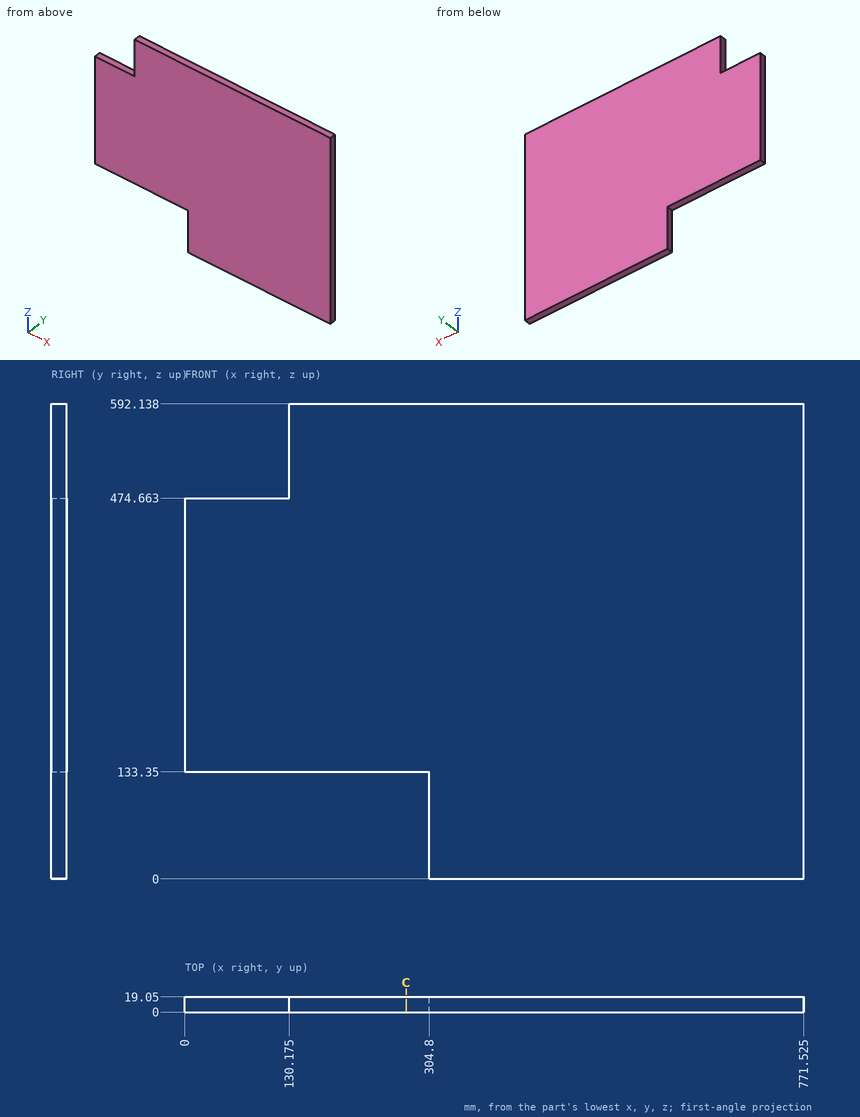
Can you work these out from the drawing? Everything is in mm from the part's minimum corner. Round coordinates to 2 decimals unless told otherwise and drop trailing zeros. Order: outer loops, then holes, each group sorted by start corner. A loop starts at its lowest first (then second) coordinate and runs counter-clockwise, first axis right, second up.
(1) I'm going to push flat-ended pins straight in: pin 1 (4 mm diameter, centred on x = 201, z = 344, fed in from -Y); pin 2 (2 mm diameter, centred on x = 109, y = 8, fed in from +Z). Where does each tip first touch, or does it pass through?
Results are:
pin 1: stops at y = 0
pin 2: stops at z = 474.66
(2) If I drill on L1, parallel to Z at x = 288.5, y = 4.75; L2, parallel to X at y = 13, z = 49 (1 decimal), over which ranges is the centre line in solid material (lowest first)?
Results are:
L1: z = 133.35 to 592.14
L2: x = 304.8 to 771.5
(3) If we section it at C-C (x = 276): Please give me the cut outline in (y, z).
Results are:
outline: (0, 133.35) - (19.05, 133.35) - (19.05, 592.14) - (0, 592.14) - close
